```python
from build123d import *


with BuildPart() as part:
    # Croquis1 → Revolución1 (revolve)
    with BuildSketch(Plane.XY, mode=Mode.PRIVATE) as revoluci_n1_sk:
        Polygon((-13, 67.989509587), (-16, 67.989509587), (-16, 31.989509587), (-13, 31.989509587), (-13, 39.989509587), (-11.5, 39.989509587), (-11.5, 59.989509587), (-13, 59.989509587), align=None)
    revolve(revoluci_n1_sk.sketch.rotate(Axis((0, 0, 0), (0, 1, 0)), 270), axis=Axis((0, 0, 0), (0, 1, 0)))


solid = part.part
```
Geometry check sheet. Reference: the model listing, model coordinates, mm. A direction names the side the tool comes from. Give positions to 0.01 mm unless a question says otherwise; leave off trailing zeros. Order: outer loops, then holes, each group sorted by start corner. A loop starts at its lowest first (then second) coordinate and runs counter-clockwise, first axis right, second up. Notation, with made-up numbers: (39, 0) - (93, 0) arc R20 cw to (93, 25) - close; hole circle Ø7 at (63, -21.75). An arc over 180 degrees is marked (long way). Answer in a Markdown table with one row per item. Add a question column.
Q1. Cross-section at D-D, the plane x = 12.5. Enter the section's corners in (y, z).
Q2. Tool access check on faces 5 (the flat face through (-13.1, 67.99, -1.3)), 6 (the cylindrical face through (7.91, 64.046, 10.316)), 7 (the cylindrical face through (7.91, 36.046, 10.316)). Record the directions out of +Z, -Z, +X, -X, +Y, -Y that give a thin tool (end or side, any length) a straight path to the whole face; none if there is none.
Q3. Cross-section at C-C, the plane y = 39.5. Enter the section's corners in (x, z), then the cut area to 3 significant figures.
Q4. Mould release check, pull along X, two halves, no side actions. Record for faces 1 (the flat face through (11, 39.99, -5)), 2 (the flat face through (-13.1, 31.99, 1.3)), 3 (the cylindrical face through (15.62, 49.74, 3.47)), 4 (the flat face through (11, 59.99, 5)): pulls with the +X half, pulls with the -X half, needs draft (parallel to the pull), parting line crosses it, or undercut.
Q5. Cross-section at A-A, the plane z = 0. Enter the section's corners in (x, y), then the cut area to 3 significant figures.
Q6. Gauge pin test, flat ends, axial feed: pin 1 (3 mm diameter, centred on y = 56, z = -2.5, fed in from -X); pin 2 (12 mm diameter, centred on y = 46, z = 12, fed in from -X); pin 3 (1 mm diameter, centred on y = 53, z = -7, fed in from -X); pin 4 (5 mm diameter, centred on y = 39, z = -1.5, fed in from +X). Record the tip position at first contact, or that the pin passes through.
Q7. Material ranges on probe 1 along X at (y, z) = (64, 0); probe 2 along X at (y, z) = (49.25, 0); probe 3 along Y at (x, z) = (-9, -8.5), recorded low to high. Write a range as from..to.
Q8. Cross-section at B-B, the plane x = 0. Enter the section's corners in (y, z), then the cut area to 3 significant figures.
Check values:
| question | item | result |
|---|---|---|
| 1 | outline | (31.99, -9.99) - (67.99, -9.99) - (67.99, -3.57) - (59.99, -3.57) - (59.99, 3.57) - (67.99, 3.57) - (67.99, 9.99) - (31.99, 9.99) - (31.99, 3.57) - (39.99, 3.57) - (39.99, -3.57) - (31.99, -3.57) - close |
| 2 | face 5 | +Z, -Z, +X, -X, +Y |
| 2 | face 6 | +Y |
| 2 | face 7 | -Y |
| 3 | outline | circle Ø32 at (0, 0); hole circle Ø26 at (0, 0) |
| 3 | area | 273 mm^2 |
| 4 | face 1 | undercut |
| 4 | face 2 | needs draft |
| 4 | face 3 | parting line crosses it |
| 4 | face 4 | undercut |
| 5 | outline | (-16, 31.99) - (-13, 31.99) - (-13, 39.99) - (-11.5, 39.99) - (-11.5, 59.99) - (-13, 59.99) - (-13, 67.99) - (-16, 67.99) - close; (11.5, 39.99) - (13, 39.99) - (13, 31.99) - (16, 31.99) - (16, 67.99) - (13, 67.99) - (13, 59.99) - (11.5, 59.99) - close |
| 5 | area | 276 mm^2 |
| 6 | pin 1 | stops at x = -15.97 |
| 6 | pin 2 | stops at x = -14.83 |
| 6 | pin 3 | stops at x = -14.62 |
| 6 | pin 4 | stops at x = 16 |
| 7 | probe 1 | x = -16..-13, 13..16 |
| 7 | probe 2 | x = -16..-11.5, 11.5..16 |
| 7 | probe 3 | y = 39.99..59.99 |
| 8 | outline | (31.99, -16) - (67.99, -16) - (67.99, -13) - (59.99, -13) - (59.99, -11.5) - (39.99, -11.5) - (39.99, -13) - (31.99, -13) - close; (31.99, 13) - (39.99, 13) - (39.99, 11.5) - (59.99, 11.5) - (59.99, 13) - (67.99, 13) - (67.99, 16) - (31.99, 16) - close |
| 8 | area | 276 mm^2 |
